Could you check a few things on this model? Use its own coordinates, in mm. A direction names the side the tool comes from. Coordinates: 2 decimals unless noted, no trailing zeros. Loops run counter-clockwise (first coordinate to the right, second up) from the corner with the lowest first, then second, coordinate; pieces in that order, holes last. Notation, with made-up numbers: (3.5, -1.5) - (17.5, -1.5) arc R15 ccw to (17.5, 16.5) - close; hole circle Ø11 at (-8.75, 61.25). An arc over 180 degrees is marked (long way). Use CSV: the item, a comma, the result in double quotes.
from build123d import *

# Parameters (mm, degrees)
SKETCH1_W           = 75
SKETCH1_H           = 3
BOSS_EXTRUDE1_DEPTH = 200
SKETCH2_R           = 4.9
BOSS_EXTRUDE2_DEPTH = 10
SKETCH3_W           = 5
SKETCH3_H           = 200
CUT_EXTRUDE1_DEPTH  = 1


with BuildPart() as part:
    # Sketch1 → Boss-Extrude1 (new body)
    with BuildSketch(Plane.XY):
        with Locations((37.5, 1.5)):
            Rectangle(SKETCH1_W, SKETCH1_H)
    extrude(amount=BOSS_EXTRUDE1_DEPTH)

    # Sketch2 → Boss-Extrude2 (add)
    with BuildSketch(Plane(origin=(0, 3, 0), x_dir=(1, 0, 0), z_dir=(0, 1, 0))):
        with Locations(Location((7.5, -10, 0), (0, 0, 90))):
            Circle(SKETCH2_R)
        with Locations(Location((47.5, -190, 0), (0, 0, 90))):
            Circle(SKETCH2_R)
    extrude(amount=BOSS_EXTRUDE2_DEPTH)

    # Sketch3 → Cut-Extrude1 (cut)
    with BuildSketch(Plane.XZ):
        with Locations((37.5, 100)):
            Rectangle(SKETCH3_W, SKETCH3_H)
    extrude(amount=-CUT_EXTRUDE1_DEPTH, mode=Mode.SUBTRACT)


solid = part.part
(1) Please list where these lines run through material, in increasing order: line 1 (Y direction, x = 32.5, z = 108.5); line 2 (Z direction, x = 7, y = 5.5); line 3 (Z direction, x = 47, y = 4).
Computed:
line 1,"y = 0 to 3"
line 2,"z = 5.13 to 14.87"
line 3,"z = 185.13 to 194.87"
(2) Will these pins go through, and if not, where does the flat tip stop? pin 1 (2.5 mm diameter, centred on x = 38, z = 144, fed in from -Y); pin 2 (6 mm diameter, centred on x = 9.5, z = 154.5, fed in from +Y); pin 3 (3 mm diameter, centred on x = 27, y = 3.5, fed in from +Z); pin 4 (1.5 mm diameter, centred on x = 11.5, y = 11.5, fed in from +Z).
Computed:
pin 1,"stops at y = 1"
pin 2,"stops at y = 3"
pin 3,"stops at z = 200"
pin 4,"stops at z = 13.67"
(3) Suppose I cut it at C-C (x = 47.5). Write out the boundary of the cut face in (y, z).
Computed:
outline,"(0, 0) - (3, 0) - (3, 185.1) - (13, 185.1) - (13, 194.9) - (3, 194.9) - (3, 200) - (0, 200) - close"
(4) Suppose I cut it at B-B (y = 8.5). Write out the boundary of the cut face in (x, z), plus the area to 3 significant figures.
Computed:
outline,"circle Ø9.8 at (7.5, 10); circle Ø9.8 at (47.5, 190)"
area,"151 mm²"
(5) Thinking about a two-plate mould opening in X: for faces 1 (the face through (37, 1, 101)), 2 (the face through (37, 3, 99)), 3 (the face through (6.028, 7.93, 5.326)), which applies, +X half, -X half, draft (parallel to the pull), parting line (faces both ways), or undercut?
Computed:
face 1,"undercut"
face 2,"draft"
face 3,"parting line"
(6) Which directions (+Z, -Z, +X, -X, +Y, -Y) give clear straight access to the entire face, cutting with the end or side of a thin tool? Please do faces 4 (the face through (46.028, 7.93, 185.326)), 5 (the face through (57, 0, 99)).
Computed:
face 4,"+Y"
face 5,"+Z, -Z, +X, -X, -Y"
(7) Suppose I cut it at D-D (z = 190). Write out the boundary of the cut face in (x, y).
Computed:
outline,"(0, 0) - (35, 0) - (35, 1) - (40, 1) - (40, 0) - (75, 0) - (75, 3) - (52.4, 3) - (52.4, 13) - (42.6, 13) - (42.6, 3) - (0, 3) - close"
(8) Suppose I cut it at A-A (z = 108). Write out the boundary of the cut face in (x, y).
Computed:
outline,"(0, 0) - (35, 0) - (35, 1) - (40, 1) - (40, 0) - (75, 0) - (75, 3) - (0, 3) - close"
